For this review, take the finished solid that the model builds, in its own axes (mm). Face numbers are marked on the shaded views. Round coordinates to 2 decimals unless told otherwise and drop trailing zeros. Order: outer loops, then holes, each group sorted by start corner. A loop starts at its lowest first (then second) coordinate and runs counter-clockwise, first axis right, second up. Notation, with made-up numbers: M 44.5,23 L 99.5,23 A13 cw 99.5,42 Z; hole C -1.5,20 d5. An arc over 180 degrees is marked long. Put each result on its own line as item: value.
from build123d import *

# Parameters (mm, degrees)
SKETCH1_R           = 25
SKETCH1_R_2         = 12.5
BOSS_EXTRUDE1_DEPTH = 4
CHAMFER1_SIZE       = 0.2


with BuildPart() as part:
    # Sketch1 → Boss-Extrude1 (new body)
    with BuildSketch(Plane(origin=(0, 0, 0), x_dir=(1, 0, 0), z_dir=(0, 1, 0))):
        with Locations(Location((0, 0, 0), (0, 0, 270))):
            Circle(SKETCH1_R)
        with BuildLine():
            ThreePointArc((0.758245274, -22.952787235), (-0.048003188, -23.74036389), (-0.841852323, -22.940290693))
            Line((-0.841852323, -22.940290693), (-0.841508405, -17.728184123))
            ThreePointArc((-0.841508405, -17.728184123), (-0.841754725, -17.708280546), (-0.841505778, -17.688377001))
            ThreePointArc((-0.841505778, -17.688377001), (-0.031775784, -16.908395573), (0.758245274, -17.708333333))
            Line((0.758245274, -17.708333333), (0.758245274, -22.927794152))
            Line((0.758245274, -22.927794152), (0.758245274, -22.952787235))
        make_face(mode=Mode.SUBTRACT)
        with BuildLine():
            ThreePointArc((-10.819733948, -20.25681947), (-11.911753925, -20.53575663), (-12.199210844, -19.445948349))
            Line((-12.199210844, -19.445948349), (-9.592859718, -14.932303611))
            ThreePointArc((-9.592859718, -14.932303611), (-9.583121248, -14.914943448), (-9.572953882, -14.897830945))
            ThreePointArc((-9.572953882, -14.897830945), (-8.481716422, -14.627212211), (-8.197506997, -15.714989162))
            Line((-8.197506997, -15.714989162), (-10.807237407, -20.235174825))
            Line((-10.807237407, -20.235174825), (-10.819733948, -20.25681947))
        make_face(mode=Mode.SUBTRACT)
        with BuildLine():
            ThreePointArc((-19.498574197, -12.133053287), (-20.583759818, -11.828609965), (-20.287800672, -10.741079849))
            Line((-20.287800672, -10.741079849), (-15.773812016, -8.135324406))
            ThreePointArc((-15.773812016, -8.135324406), (-15.756698172, -8.125159298), (-15.739336724, -8.115423119))
            ThreePointArc((-15.739336724, -8.115423119), (-14.658987995, -8.42667915), (-14.956743889, -9.510826336))
            Line((-14.956743889, -9.510826336), (-19.476929551, -12.120556745))
            Line((-19.476929551, -12.120556745), (-19.498574197, -12.133053287))
        make_face(mode=Mode.SUBTRACT)
        with BuildLine():
            ThreePointArc((12.133053287, -19.498574197), (11.828609965, -20.583759818), (10.741079849, -20.287800672))
            Line((10.741079849, -20.287800672), (8.135324406, -15.773812016))
            ThreePointArc((8.135324406, -15.773812016), (8.125159298, -15.756698172), (8.115423119, -15.739336724))
            ThreePointArc((8.115423119, -15.739336724), (8.42667915, -14.658987995), (9.510826336, -14.956743889))
            Line((9.510826336, -14.956743889), (12.120556745, -19.476929551))
            Line((12.120556745, -19.476929551), (12.133053287, -19.498574197))
        make_face(mode=Mode.SUBTRACT)
        with BuildLine():
            ThreePointArc((20.25681947, -10.819733948), (20.53575663, -11.911753925), (19.445948349, -12.199210844))
            Line((19.445948349, -12.199210844), (14.932303611, -9.592859718))
            ThreePointArc((14.932303611, -9.592859718), (14.914943448, -9.583121248), (14.897830945, -9.572953882))
            ThreePointArc((14.897830945, -9.572953882), (14.627212211, -8.481716422), (15.714989162, -8.197506997))
            Line((15.714989162, -8.197506997), (20.235174825, -10.807237407))
            Line((20.235174825, -10.807237407), (20.25681947, -10.819733948))
        make_face(mode=Mode.SUBTRACT)
        with BuildLine():
            ThreePointArc((22.952787235, 0.758245274), (23.74036389, -0.048003188), (22.940290693, -0.841852323))
            Line((22.940290693, -0.841852323), (17.728184123, -0.841508405))
            ThreePointArc((17.728184123, -0.841508405), (17.708280546, -0.841754725), (17.688377001, -0.841505778))
            ThreePointArc((17.688377001, -0.841505778), (16.908395573, -0.031775784), (17.708333333, 0.758245274))
            Line((17.708333333, 0.758245274), (22.927794152, 0.758245274))
            Line((22.927794152, 0.758245274), (22.952787235, 0.758245274))
        make_face(mode=Mode.SUBTRACT)
        with BuildLine():
            ThreePointArc((-22.952787235, -0.758245274), (-23.74036389, 0.048003188), (-22.940290693, 0.841852323))
            Line((-22.940290693, 0.841852323), (-17.728184123, 0.841508405))
            ThreePointArc((-17.728184123, 0.841508405), (-17.708280546, 0.841754725), (-17.688377001, 0.841505778))
            ThreePointArc((-17.688377001, 0.841505778), (-16.908395573, 0.031775784), (-17.708333333, -0.758245274))
            Line((-17.708333333, -0.758245274), (-22.927794152, -0.758245274))
            Line((-22.927794152, -0.758245274), (-22.952787235, -0.758245274))
        make_face(mode=Mode.SUBTRACT)
        with BuildLine():
            ThreePointArc((-20.25681947, 10.819733948), (-20.53575663, 11.911753925), (-19.445948349, 12.199210844))
            Line((-19.445948349, 12.199210844), (-14.932303611, 9.592859718))
            ThreePointArc((-14.932303611, 9.592859718), (-14.914943448, 9.583121248), (-14.897830945, 9.572953882))
            ThreePointArc((-14.897830945, 9.572953882), (-14.627212211, 8.481716422), (-15.714989162, 8.197506997))
            Line((-15.714989162, 8.197506997), (-20.235174825, 10.807237407))
            Line((-20.235174825, 10.807237407), (-20.25681947, 10.819733948))
        make_face(mode=Mode.SUBTRACT)
        with Locations(Location((0, 0, 0), (0, 0, 270))):
            Circle(SKETCH1_R_2, mode=Mode.SUBTRACT)
        with BuildLine():
            ThreePointArc((-12.133053287, 19.498574197), (-11.828609965, 20.583759818), (-10.741079849, 20.287800672))
            Line((-10.741079849, 20.287800672), (-8.135324406, 15.773812016))
            ThreePointArc((-8.135324406, 15.773812016), (-8.125159298, 15.756698172), (-8.115423119, 15.739336724))
            ThreePointArc((-8.115423119, 15.739336724), (-8.42667915, 14.658987995), (-9.510826336, 14.956743889))
            Line((-9.510826336, 14.956743889), (-12.120556745, 19.476929551))
            Line((-12.120556745, 19.476929551), (-12.133053287, 19.498574197))
        make_face(mode=Mode.SUBTRACT)
        with BuildLine():
            ThreePointArc((19.498574197, 12.133053287), (20.583759818, 11.828609965), (20.287800672, 10.741079849))
            Line((20.287800672, 10.741079849), (15.773812016, 8.135324406))
            ThreePointArc((15.773812016, 8.135324406), (15.756698172, 8.125159298), (15.739336724, 8.115423119))
            ThreePointArc((15.739336724, 8.115423119), (14.658987995, 8.42667915), (14.956743889, 9.510826336))
            Line((14.956743889, 9.510826336), (19.476929551, 12.120556745))
            Line((19.476929551, 12.120556745), (19.498574197, 12.133053287))
        make_face(mode=Mode.SUBTRACT)
        with BuildLine():
            ThreePointArc((10.819733948, 20.25681947), (11.911753925, 20.53575663), (12.199210844, 19.445948349))
            Line((12.199210844, 19.445948349), (9.592859718, 14.932303611))
            ThreePointArc((9.592859718, 14.932303611), (9.583121248, 14.914943448), (9.572953882, 14.897830945))
            ThreePointArc((9.572953882, 14.897830945), (8.481716422, 14.627212211), (8.197506997, 15.714989162))
            Line((8.197506997, 15.714989162), (10.807237407, 20.235174825))
            Line((10.807237407, 20.235174825), (10.819733948, 20.25681947))
        make_face(mode=Mode.SUBTRACT)
        with BuildLine():
            ThreePointArc((0.841505778, 17.688377001), (0.031775784, 16.908395573), (-0.758245274, 17.708333333))
            Line((-0.758245274, 17.708333333), (-0.758245274, 22.927794152))
            Line((-0.758245274, 22.927794152), (-0.758245274, 22.952787235))
            ThreePointArc((-0.758245274, 22.952787235), (0.048003188, 23.74036389), (0.841852323, 22.940290693))
            Line((0.841852323, 22.940290693), (0.841508405, 17.728184123))
            ThreePointArc((0.841508405, 17.728184123), (0.841754725, 17.708280546), (0.841505778, 17.688377001))
        make_face(mode=Mode.SUBTRACT)
    extrude(amount=BOSS_EXTRUDE1_DEPTH)

    # Chamfer1
    chamfer1_edges = [part.edges().sort_by_distance(p)[0] for p in [
        (0, 4, -12.5),
        (0, 4, -25),
        (0, 0, -25),
        (0, 0, -12.5),
    ]]
    chamfer(chamfer1_edges, length=CHAMFER1_SIZE)


solid = part.part
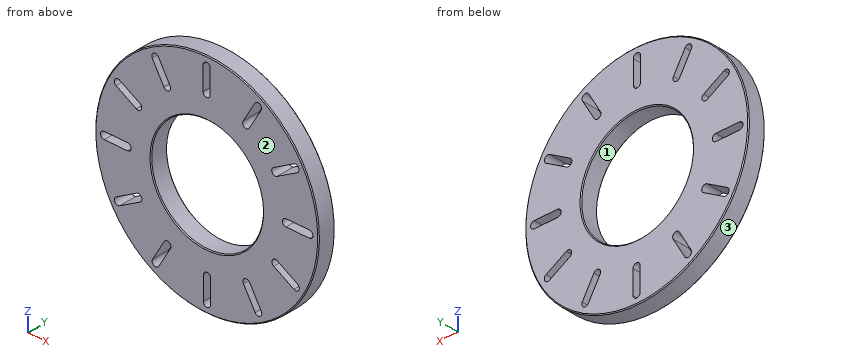
(1) Draft analysis for pull direction Z (two halves, no side actions). For the marked faces 1, 2 and 3, state which applies: released by +Z, released by -Z, zero draft, split by the parting line, or undercut.
A:
face 1: undercut
face 2: zero draft
face 3: split by the parting line
(2) Insertion check: pin 1 Ø2 at (x, y) = (19.5, 1.5) entering from +Z; pin 2 Ø1.2 at (x, y) = (-20, 2) entering from +Z; pin 3 Ø1.2 at (y, z) = (3, 19.5) entering from -X. Each pin has a flat end and moves straight along its axis. Give the tip position at first contact, or say it passes through.
A:
pin 1: stops at z = 16.82
pin 2: stops at z = 15.77
pin 3: stops at x = -16.36
(3) Add section B-B on z = 0. Give the boundary of the cut face in (x, y), then the cut area to 3 significant figures.
A:
outline: M -25,0.2 L -24.8,0 L -23.74,0 L -23.74,4 L -24.8,4 L -25,3.8 Z; M -16.91,0 L -12.7,0 L -12.5,0.2 L -12.5,3.8 L -12.7,4 L -16.91,4 Z; M 12.5,0.2 L 12.7,0 L 16.91,0 L 16.91,4 L 12.7,4 L 12.5,3.8 Z; M 23.74,0 L 24.8,0 L 25,0.2 L 25,3.8 L 24.8,4 L 23.74,4 Z
area: 45.2 mm2
(4) Add section A-A on y = 1.7. State how many separate pieces and enclosed holes the cut face has, then the cut area to 3 significant figures.
A:
separate pieces: 1
enclosed holes: 13
area: 1,350 mm2
(5) To check wall thickness, follow L1, parallel to X at y = 2.8, z = 0; L2, parallel to Z at x = -18.5, y = 1.6; L3, parallel to Z at x = -9, y = 2.55. State the ranges of each line that lie inside material, in increasing order.
A:
L1: x = -25 to -23.74, -16.91 to -12.5, 12.5 to 16.91, 23.74 to 25
L2: z = -16.82 to -11.65, -9.81 to -0.84, 0.76 to 9.71, 11.56 to 16.82
L3: z = -23.32 to -17.27, -14.58 to -8.67, 8.67 to 14.52, 17.1 to 23.32
(6) Add section C-C on x = 0. Give the boundary of the cut face in (y, z), then the cut area to 3 significant figures.
A:
outline: M 0,-24.8 L 0.2,-25 L 3.8,-25 L 4,-24.8 L 4,-23.74 L 0,-23.74 Z; M 0,-16.91 L 4,-16.91 L 4,-12.7 L 3.8,-12.5 L 0.2,-12.5 L 0,-12.7 Z; M 0,12.7 L 0.2,12.5 L 3.8,12.5 L 4,12.7 L 4,16.91 L 0,16.91 Z; M 0,23.74 L 4,23.74 L 4,24.8 L 3.8,25 L 0.2,25 L 0,24.8 Z
area: 45.2 mm2
